```python
from build123d import *

# Parameters (mm, degrees)
SKETCH1_R           = 2.032
BOSS_EXTRUDE1_DEPTH = 304.8
SKETCH2_W           = 42.88308167
SKETCH2_H           = 34.457496419
CUT_EXTRUDE1_DEPTH  = 400


with BuildPart() as part:
    # Sketch1 → Boss-Extrude1 (new body, symmetric)
    with BuildSketch(Plane.XY):
        with BuildLine():
            Line((-12.7, 10.591838253), (-12.7, 2.108161747))
            ThreePointArc((-12.7, 2.108161747), (-12.078025605, 0.612955845), (-10.5791, 0))
            ThreePointArc((-10.5791, 0), (-10.06475, 0.508039196), (-9.5504, 0))
            Line((-9.5504, 0), (-6.3246, 0))
            ThreePointArc((-6.3246, 0), (-5.8166, 0.508), (-5.3086, 0))
            Line((-5.3086, 0), (5.3086, 0))
            ThreePointArc((5.3086, 0), (5.8166, 0.508), (6.3246, 0))
            Line((6.3246, 0), (9.5504, 0))
            ThreePointArc((9.5504, 0), (10.06475, 0.508039196), (10.5791, 0))
            ThreePointArc((10.5791, 0), (12.078025605, 0.612955845), (12.7, 2.108161747))
            Line((12.7, 2.108161747), (12.7, 10.591838253))
            ThreePointArc((12.7, 10.591838253), (12.078025605, 12.087044155), (10.5791, 12.7))
            ThreePointArc((10.5791, 12.7), (10.06475, 12.191960804), (9.5504, 12.7))
            Line((9.5504, 12.7), (6.3246, 12.7))
            ThreePointArc((6.3246, 12.7), (5.816599999, 12.191999983), (5.3086, 12.700000002))
            Line((5.3086, 12.700000002), (4.302307889, 12.700000002))
            ThreePointArc((4.302307889, 12.700000002), (3.197407889, 11.595100002), (4.302307889, 10.490200002))
            Line((4.302307889, 10.490200002), (6.487959021, 10.490200002))
            ThreePointArc((6.487959021, 10.490200002), (7.426620626, 9.863006369), (7.20637951, 8.755779512))
            Line((7.20637951, 8.755779512), (3.87633597, 5.425735971))
            ThreePointArc((3.87633597, 5.425735971), (2.846291837, 4.737482486), (1.631271939, 4.495800002))
            Line((1.631271939, 4.495800002), (-1.631271939, 4.495800002))
            ThreePointArc((-1.631271939, 4.495800002), (-2.846291837, 4.737482486), (-3.87633597, 5.425735971))
            Line((-3.87633597, 5.425735971), (-7.20637951, 8.755779512))
            ThreePointArc((-7.20637951, 8.755779512), (-7.426620626, 9.863006369), (-6.487959021, 10.490200002))
            Line((-6.487959021, 10.490200002), (-4.302307889, 10.490200002))
            ThreePointArc((-4.302307889, 10.490200002), (-3.197407889, 11.595100002), (-4.302307889, 12.700000002))
            Line((-4.302307889, 12.700000002), (-5.3086, 12.700000002))
            ThreePointArc((-5.3086, 12.700000002), (-5.816599999, 12.191999985), (-6.3246, 12.7))
            Line((-6.3246, 12.7), (-9.5504, 12.7))
            ThreePointArc((-9.5504, 12.7), (-10.06475, 12.191960804), (-10.5791, 12.7))
            ThreePointArc((-10.5791, 12.7), (-12.078025605, 12.087044155), (-12.7, 10.591838253))
        make_face()
        with Locations((-8.73125, 3.9624)):
            Circle(SKETCH1_R, mode=Mode.SUBTRACT)
        with Locations((8.73125, 3.9624)):
            Circle(SKETCH1_R, mode=Mode.SUBTRACT)
    extrude(amount=BOSS_EXTRUDE1_DEPTH, both=True)

    # Sketch2 → Cut-Extrude1 (cut)
    with BuildSketch(Plane(origin=(0, 0, -304.8), x_dir=(-1, 0, 0), z_dir=(0, 0, -1))):
        with Locations((2.724035754, 4.894294136)):
            Rectangle(SKETCH2_W, SKETCH2_H)
    extrude(amount=-CUT_EXTRUDE1_DEPTH, mode=Mode.SUBTRACT)


solid = part.part
```
For this review, take the finished solid that the model builds, in its own axes (mm). A direction names the side the tool comes from. Round coordinates to 2 decimals unless told otherwise and drop trailing zeros. One line per question, with ' | ' between items. Start each with the question number.
(1) Mouldability with a two-part tool opening along Y and no side actions: class faces 1 (the face through (-5.52, 7.07, 201.47)), 2 (the face through (-8, 0, 201)), 3 (the face through (0, 4.496, 201)), 4 (the face through (12.7, 6, 201)) as released by +Y, released by -Y, zero draft, split by the parting line, or undercut.
(2) Insertion check: P1, Ø2.5, axis at x = 0.5, z = 215.5, coming from the +Y side. The pin has a flat end and moves straight along its axis. Give the tip position at first contact, or say it passes through.
(3) For line 1 along X through (y, z) = (3, 114); line 2 along X through (y, z) = (5.75, 184); line 3 along X through (y, z) = (3.5, 155), list the stretches that pass through material, from the lowest coordinate up. Write a range as from..to.
(4) Add section A-A, the plane z = 278.5. Give the number of separate pieces and of enclosed holes in the cut face, plus the area to 3 significant figures.
(5) Tool access review of faces 5 (the face through (8, 12.7, 201)), 6 (the face through (5.56, 7.11, 201.47)): name each direction out of +Z, -Z, +X, -X, +Y, -Y from which nothing blocks a thin tool from reaching the whole face with its end or side.
Answer list:
1) face 1: undercut | face 2: released by -Y | face 3: released by +Y | face 4: zero draft
2) P1: y = 4.5
3) line 1: -12.7..-10.52, -6.94..6.94, 10.52..12.7 | line 2: -12.7..-9.7, -7.77..-4.2, 4.2..7.77, 9.7..12.7 | line 3: -12.7..-10.71, -6.75..6.75, 10.71..12.7
4) separate pieces: 1 | enclosed holes: 2 | area: 206 mm²
5) face 5: +Z, -Z, +X, -X, +Y | face 6: +Z, -Z
